from build123d import *


with BuildPart() as part:
    # Sketch1 → Revolve1 (revolve)
    with BuildSketch(Plane(origin=(0, 0, 0), x_dir=(0, 0, -1), z_dir=(1, 0, 0))):
        Polygon((-3, 0), (-3, -1.5), (-2.6, -1.5), (-2.6, -1.3), (-2.5, -1.3), (-2.5, -1.4), (-1.5, -1.4), (-1.5, -1.3), (-1.4, -1.3), (-1.4, -1.5), (-1, -1.5), (-1, 0), align=None)
    revolve1 = revolve(axis=Axis((0, 0, 0), (0, -1, 0)))

    # Mirror1: Revolve1 across plane
    add(revolve1.mirror(Plane(origin=(0, 0, 1), x_dir=(0, 0, 1), z_dir=(0, 1, 0))))


solid = part.part
Design review of the part built by this model. Coordinates are the model's own, in mm. Give positions to 0.01 mm unless a question says otherwise; leave off trailing zeros. Loops run counter-clockwise (first coordinate to the right, second up) from the corner with the lowest first, then second, coordinate; pieces in that order, holes last. Notation, with made-up numbers: M 68.5,-28 L 124.5,-28 A14 ccw 124.5,-19 Z; hole C 65,-34 d2. An arc over 180 degrees is marked long. One line per question, with ' | ' between items. Start each with the question number.
1. Insertion check: P1, Ø1, axis at y = 0, z = 1, coming from the -X side; P2, Ø1.2, axis at x = 0, z = 0, coming from the -Y side. Each pin has a flat end and moves straight along its axis. Give the tip position at first contact, or say it passes through.
2. The part is to be moulded in two halves that separate along Z. For faces 1 (the face through (0, -1.4, 2)), 2 (the face through (0, 0, -3)), say which applies: released by +Z, released by -Z, zero draft, split by the parting line, or undercut.
3. Add section A-A (y = 0). Write out the cut boundary in (x, z).
4. Add section C-C (z = 2.15). Write out the cut boundary in (x, y), plus the area to 3 significant figures.
5. Add section B-B (x = -1.7). Write out the cut boundary in (y, z), plus the area to 3 significant figures.
6. To check wall thickness, follow L1, parallel to X at y = 1.45, z = 0; L2, parallel to X at y = 0.85, z = 0; L3, parallel to Y at x = -1.85, z = -0.1. State the ranges of each line that lie inside material, in increasing order.
Worked out:
1) P1: stops at x = -2.96 | P2: passes through
2) face 1: undercut | face 2: split by the parting line
3) outline: C 0,0 d6; hole C 0,0 d2
4) outline: M -2.09,-1.5 L -1.46,-1.5 L -1.46,-1.3 L -1.28,-1.3 L -1.28,-1.4 L 1.28,-1.4 L 1.28,-1.3 L 1.46,-1.3 L 1.46,-1.5 L 2.09,-1.5 L 2.09,1.5 L 1.46,1.5 L 1.46,1.3 L 1.28,1.3 L 1.28,1.4 L -1.28,1.4 L -1.28,1.3 L -1.46,1.3 L -1.46,1.5 L -2.09,1.5 Z | area: 11.9 mm²
5) outline: M -1.5,-2.47 L 1.5,-2.47 L 1.5,-1.97 L 1.3,-1.97 L 1.3,-1.83 L 1.4,-1.83 L 1.4,1.83 L 1.3,1.83 L 1.3,1.97 L 1.5,1.97 L 1.5,2.47 L -1.5,2.47 L -1.5,1.97 L -1.3,1.97 L -1.3,1.83 L -1.4,1.83 L -1.4,-1.83 L -1.3,-1.83 L -1.3,-1.97 L -1.5,-1.97 Z | area: 14.0 mm²
6) L1: x = -3 to -2.6, -1.4 to -1, 1 to 1.4, 2.6 to 3 | L2: x = -3 to -1, 1 to 3 | L3: y = -1.4 to 1.4
